Can you work these out from the model? Positions are in its coordinate system, mm. A direction names the side the tool comes from. Coordinates: 2 decimals unless noted, no trailing zeros. Order: outer loops, then holes, each group sorted by start corner. A loop starts at its lowest first (then second) coordinate and runs counter-clockwise, first axis right, second up. Notation, with made-up numbers: (82.5, 38.5) -> (134.5, 38.5) arc R31 ccw to (134.5, 65.5) -> close; hole circle Ø5 at (-35.75, -16). An arc over 180 degrees is marked (long way). Write item = value, one per line.
```python
from build123d import *

# Parameters (mm, degrees)
F1_DEPTH       = 82.55
F2_R           = 7.62
F3_R           = 2.54
F6_D           = 4.826
F6_DEPTH       = 12.7
F6_TIP         = 1.4498766737
F6_ON_F5_D     = 4.826
F6_ON_F5_DEPTH = 12.7
F6_ON_F5_TIP   = 1.4498766737
F8_D           = 4.826
F8_CBORE_D     = 9.4742
F8_CBORE_DEPTH = 3.3782


with BuildPart() as f1:
    # F0 (on Front) → F1 (new body)
    with BuildSketch(Plane.XZ):
        Polygon((0, 88.9), (0, 0), (88.2142, 0), (88.2142, 9.7282), (44.1071, 9.7282), (44.1071, 88.9), align=None)
    extrude(amount=F1_DEPTH)

    # F2
    f2_edges = [f1.edges().sort_by_distance(p)[0] for p in [
        (44.1071, -41.275, 9.7282),
    ]]
    fillet(f2_edges, radius=F2_R)

    # F3
    f3_edges = [f1.edges().sort_by_distance(p)[0] for p in [
        (44.1071, -41.275, 88.9),
        (0, -41.275, 88.9),
        (0, -41.275, 0),
        (88.2142, -41.275, 9.7282),
        (88.2142, -41.275, 0),
        (22.05355, 0, 88.9),
        (22.05355, -82.55, 88.9),
        (44.1071, -82.55, 53.1241),
        (69.97065, -82.55, 9.7282),
        (69.97065, 0, 9.7282),
        (44.1071, 0, 53.1241),
        (0, 0, 44.45),
        (44.1071, 0, 0),
        (0, -82.55, 44.45),
        (44.1071, -82.55, 0),
        (88.2142, -82.55, 4.8641),
        (88.2142, 0, 4.8641),
    ]]
    fillet(f3_edges, radius=F3_R)

    # F6
    with Locations(Plane.XY.offset(88.9)):
        with Locations((25.4, -7.9375), (25.4, -74.6125)):
            Hole(F6_D / 2, depth=F6_DEPTH)
            with Locations((0, 0, -(F6_DEPTH + F6_TIP / 2))):  # 118° drill point
                Cone(0, F6_D / 2, F6_TIP, mode=Mode.SUBTRACT)

    # F6 on F5
    with Locations(Plane(origin=(0, 0, 0), x_dir=(1, 0, 0), z_dir=(0, 0, -1))):
        with Locations((20.32, 69.85), (20.32, 12.7)):
            Hole(F6_ON_F5_D / 2, depth=F6_ON_F5_DEPTH)
            with Locations((0, 0, -(F6_ON_F5_DEPTH + F6_ON_F5_TIP / 2))):  # 118° drill point
                Cone(0, F6_ON_F5_D / 2, F6_ON_F5_TIP, mode=Mode.SUBTRACT)

    # F8 (through all)
    with Locations(Plane.XY.offset(9.7282)):
        with Locations((78.0542, -12.7), (78.0542, -69.85)):
            CounterBoreHole(F8_D / 2, F8_CBORE_D / 2, F8_CBORE_DEPTH)


solid = f1.part
```
Item 1: For faces 4 (the cylindrical face through (43.38, -0.76, 52.34)), 5 (the cylindrical face through (25.71, -72.22, 82.46)), 6 (the cylindrical face through (68.46, -81.83, 8.96)), 7 (the cylindrical face through (20.843, -67.494, 6.439)), which set-ups out of +Z, -Z, +X, -X, +Y, -Y let a thin tool reach every point of the face, with its end or its side?
A:
face_4 = +Z, +X, +Y
face_5 = +Z
face_6 = +Z, +X, -Y
face_7 = -Z
Item 2: I'm going to push flat-ended pins straight in: P1, Ø8, axis at x = 79, y = -28.5, coming from the +Z side; P2, Ø20.5, axis at y = -26.5, z = 48.5, coming from the +X side; P3, Ø8.5, axis at x = 78.05, y = -69.85, coming from the +Z side. Where does each tip first touch, or does it pass through?
A:
P1 = 9.73
P2 = 44.11
P3 = 6.35
Item 3: I want a section at B-B, the plane y = -39.5. Please give me the cut outline in (x, z), plus the area to 3 significant figures.
A:
outline = (0, 2.54) arc R2.54 ccw to (2.54, 0) -> (85.67, 0) arc R2.54 ccw to (88.21, 2.54) -> (88.21, 7.19) arc R2.54 ccw to (85.67, 9.73) -> (51.73, 9.73) arc R7.62 cw to (44.11, 17.35) -> (44.11, 86.36) arc R2.54 ccw to (41.57, 88.9) -> (2.54, 88.9) arc R2.54 ccw to (0, 86.36) -> close
area = 4,360 mm2
Item 4: If we mould it in two halves opening along X, with no side actions, what happens to faces 1 (the cylindrical face through (0.764, -41.817, 0.724)), 2 (the conical face through (25.31, -75.02, 75)), 3 (the cylindrical face through (43.38, -41.82, 88.14))? For each: pulls with the +X half, pulls with the -X half, needs draft (parallel to the pull), parting line crosses it, or undercut.
A:
face_1 = pulls with the -X half
face_2 = undercut
face_3 = pulls with the +X half
Item 5: If I drill on probe 1 along Y at (x, z) = (25.4, 79.75); probe 2 along Y at (x, z) = (20.32, 6.75); probe 3 along X at (y, z) = (-61, 17), over which ranges is the centre line in solid material (lowest first)?
A:
probe_1 = -82.55 to -77.03, -72.2 to -10.35, -5.52 to 0
probe_2 = -82.55 to -72.26, -67.44 to -15.11, -10.29 to 0
probe_3 = 0 to 44.12
Item 6: I want a section at C-C, the plane z = 27.5. Please give me the cut outline in (x, y).
A:
outline = (0, -80.01) arc R2.54 ccw to (2.54, -82.55) -> (41.57, -82.55) arc R2.54 ccw to (44.11, -80.01) -> (44.11, -2.54) arc R2.54 ccw to (41.57, 0) -> (2.54, 0) arc R2.54 ccw to (0, -2.54) -> close
Item 7: I want a section at A-A, the plane x = 78.5. Please give me the cut outline in (y, z).
A:
outline = (-82.55, 2.54) arc R2.54 ccw to (-80.01, 0) -> (-72.22, 0) -> (-72.22, 6.35) -> (-74.57, 6.35) -> (-74.57, 9.73) -> (-80.01, 9.73) arc R2.54 ccw to (-82.55, 7.19) -> close; (-67.48, 0) -> (-15.07, 0) -> (-15.07, 6.35) -> (-17.42, 6.35) -> (-17.42, 9.73) -> (-65.13, 9.73) -> (-65.13, 6.35) -> (-67.48, 6.35) -> close; (-10.33, 0) -> (-2.54, 0) arc R2.54 ccw to (0, 2.54) -> (0, 7.19) arc R2.54 ccw to (-2.54, 9.73) -> (-7.98, 9.73) -> (-7.98, 6.35) -> (-10.33, 6.35) -> close
Item 8: I want a section at D-D, the plane x = 65. Please give me the cut outline in (y, z).
A:
outline = (-82.55, 2.54) arc R2.54 ccw to (-80.01, 0) -> (-2.54, 0) arc R2.54 ccw to (0, 2.54) -> (0, 7.19) arc R2.54 ccw to (-2.54, 9.73) -> (-80.01, 9.73) arc R2.54 ccw to (-82.55, 7.19) -> close
